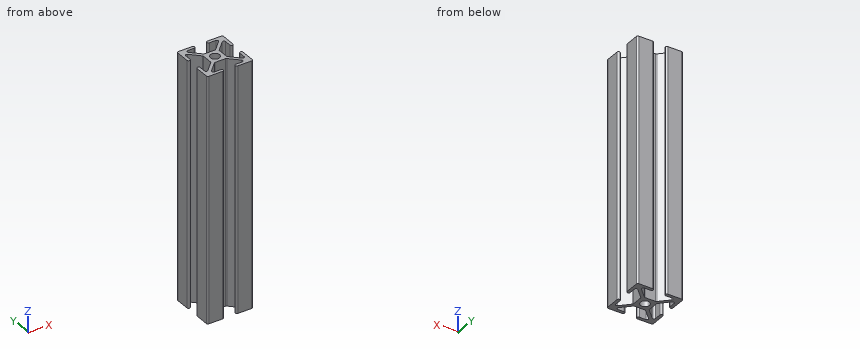
```python
from build123d import *

# Parameters (mm, degrees)
SALIENTE_EXTRUIR1_DEPTH = 190
CROQUIS2_R              = 3
CORTAR_EXTRUIR1_DEPTH   = 192.180542943
CORTAR_EXTRUIR3_DEPTH   = 192.180542943
CROQUIS4_W              = 33.127581221
CROQUIS4_H              = 30
CORTAR_EXTRUIR4_DEPTH   = 38


with BuildPart() as part:
    # Croquis1 → Saliente-Extruir1 (new body)
    with BuildSketch(Plane.XY):
        with BuildLine():
            Line((-14, 15), (14, 15))
            ThreePointArc((14, 15), (14.707106781, 14.707106781), (15, 14))
            Line((15, 14), (15, -14))
            ThreePointArc((15, -14), (14.707106781, -14.707106781), (14, -15))
            Line((14, -15), (-14, -15))
            ThreePointArc((-14, -15), (-14.707106781, -14.707106781), (-15, -14))
            Line((-15, -14), (-15, 14))
            ThreePointArc((-15, 14), (-14.707106781, 14.707106781), (-14, 15))
        make_face()
    extrude(amount=-SALIENTE_EXTRUIR1_DEPTH)

    # Croquis2 → Cortar-Extruir1 (cut, through all)
    with BuildSketch(Plane.XY):
        Circle(CROQUIS2_R)
    extrude(amount=-CORTAR_EXTRUIR1_DEPTH, mode=Mode.SUBTRACT)

    # Croquis3 → Cortar-Extruir3 (cut, through all)
    with BuildSketch(Plane.XY):
        with BuildLine():
            Line((-5.492893219, 4.078679656), (-11.292893219, 9.878679656))
            ThreePointArc((-11.292893219, 9.878679656), (-12.382683432, 10.095452408), (-13, 9.171572875))
            Line((-13, 9.171572875), (-13, 5))
            ThreePointArc((-13, 5), (-14, 4), (-15, 5))
            Line((-15, 5), (-15, -5))
            ThreePointArc((-15, -5), (-14, -4), (-13, -5))
            Line((-13, -5), (-13, -9.171572875))
            ThreePointArc((-13, -9.171572875), (-12.382683432, -10.095452408), (-11.292893219, -9.878679656))
            Line((-11.292893219, -9.878679656), (-5.492893219, -4.078679656))
            ThreePointArc((-5.492893219, -4.078679656), (-5.276120467, -3.754256308), (-5.2, -3.371572875))
            Line((-5.2, -3.371572875), (-5.2, 3.371572875))
            ThreePointArc((-5.2, 3.371572875), (-5.276120467, 3.754256308), (-5.492893219, 4.078679656))
        make_face()
        with BuildLine():
            ThreePointArc((-9.171572875, 13), (-10.095452408, 12.382683432), (-9.878679656, 11.292893219))
            Line((-9.878679656, 11.292893219), (-4.078679656, 5.492893219))
            ThreePointArc((-4.078679656, 5.492893219), (-3.754256308, 5.276120467), (-3.371572875, 5.2))
            Line((-3.371572875, 5.2), (3.371572875, 5.2))
            ThreePointArc((3.371572875, 5.2), (3.754256308, 5.276120467), (4.078679656, 5.492893219))
            Line((4.078679656, 5.492893219), (9.878679656, 11.292893219))
            ThreePointArc((9.878679656, 11.292893219), (10.095452408, 12.382683432), (9.171572875, 13))
            Line((9.171572875, 13), (5, 13))
            ThreePointArc((5, 13), (4, 14), (5, 15))
            Line((5, 15), (-5, 15))
            ThreePointArc((-5, 15), (-4.292893219, 14.707106781), (-4, 14))
            ThreePointArc((-4, 14), (-4.292893219, 13.292893219), (-5, 13))
            Line((-5, 13), (-9.171572875, 13))
        make_face()
        with BuildLine():
            Line((9.878679656, -11.292893219), (4.078679656, -5.492893219))
            ThreePointArc((4.078679656, -5.492893219), (3.754256308, -5.276120467), (3.371572875, -5.2))
            Line((3.371572875, -5.2), (-3.371572875, -5.2))
            ThreePointArc((-3.371572875, -5.2), (-3.754256308, -5.276120467), (-4.078679656, -5.492893219))
            Line((-4.078679656, -5.492893219), (-9.878679656, -11.292893219))
            ThreePointArc((-9.878679656, -11.292893219), (-10.095452408, -12.382683432), (-9.171572875, -13))
            Line((-9.171572875, -13), (-5, -13))
            ThreePointArc((-5, -13), (-4.292893219, -13.292893219), (-4, -14))
            ThreePointArc((-4, -14), (-4.292893219, -14.707106781), (-5, -15))
            Line((-5, -15), (5, -15))
            ThreePointArc((5, -15), (4, -14), (5, -13))
            Line((5, -13), (9.171572875, -13))
            ThreePointArc((9.171572875, -13), (10.095452408, -12.382683432), (9.878679656, -11.292893219))
        make_face()
        with BuildLine():
            ThreePointArc((13, 9.171572875), (12.382683432, 10.095452408), (11.292893219, 9.878679656))
            Line((11.292893219, 9.878679656), (5.492893219, 4.078679656))
            ThreePointArc((5.492893219, 4.078679656), (5.276120467, 3.754256308), (5.2, 3.371572875))
            Line((5.2, 3.371572875), (5.2, -3.371572875))
            ThreePointArc((5.2, -3.371572875), (5.276120467, -3.754256308), (5.492893219, -4.078679656))
            Line((5.492893219, -4.078679656), (11.292893219, -9.878679656))
            ThreePointArc((11.292893219, -9.878679656), (12.382683432, -10.095452408), (13, -9.171572875))
            Line((13, -9.171572875), (13, -5))
            ThreePointArc((13, -5), (14, -4), (15, -5))
            Line((15, -5), (15, 5))
            ThreePointArc((15, 5), (14, 4), (13, 5))
            Line((13, 5), (13, 9.171572875))
        make_face()
    extrude(amount=-CORTAR_EXTRUIR3_DEPTH, mode=Mode.SUBTRACT)

    # Croquis4 → Cortar-Extruir4 (cut)
    with BuildSketch(Plane(origin=(0, 15, 0), x_dir=(1, 0, 0), z_dir=(0, 1, 0))):
        with Locations((-1.56379061, 15)):
            Rectangle(CROQUIS4_W, CROQUIS4_H)
    extrude(amount=-CORTAR_EXTRUIR4_DEPTH, mode=Mode.SUBTRACT)


solid = part.part
```
The model under review builds one solid part; all positions refer to its coordinate system, in mm. Round coordinates to 2 decimals unless told otherwise and drop trailing zeros. Loops run counter-clockwise (first coordinate to the right, second up) from the corner with the lowest first, then second, coordinate; pieces in that order, holes last. Notation, with made-up numbers: (-8, 62) -> (-4, 62) arc R29 ccw to (-4, 94) -> close; hole circle Ø4 at (-29.75, -9). An arc over 180 degrees is marked (long way). Answer as a JSON object with one key per item and string values. Group by question number.
1) We need section C-C on y = -7. Write out the cut boundary in (x, z), then the cut area to 3 significant figures.
2) For line 1 (Y direction, x = 6, z = -95); line 2 (X direction, y = -9.5, z = -133.5); line 3 (Y direction, x = 0, z = -104), list the stretches that pass through material, from the lowest coordinate up. Write a range as [from, to].
3) For pin 1 Ø7.5 at (y, z) = (-0.5, -128.5) entering from -X; pin 2 Ø2 at (x, z) = (0, -124) entering from +Y; pin 3 Ø5.5 at (y, z) = (1, -128.5) entering from +X, all flat-tipped, find the tip position at first contact; note any pin that passes through.
4) We need section A-A on y = 0. Write out the cut boundary in (x, z).
Result set:
{
 "1": {"outline": "(-15, -190) -> (-13, -190) -> (-13, -30) -> (-15, -30) -> close; (-8.41, -190) -> (-5.59, -190) -> (-5.59, -30) -> (-8.41, -30) -> close; (5.59, -190) -> (8.41, -190) -> (8.41, -30) -> (5.59, -30) -> close; (13, -190) -> (15, -190) -> (15, -30) -> (13, -30) -> close", "area": "1,550 mm²"},
 "2": {"line 1": "[-15, -13], [-7.41, -4.59], [4.59, 7.41], [13, 15]", "line 2": "[-15, -12.94], [-10.91, -8.09], [8.09, 10.91], [12.94, 15]", "line 3": "[-5.2, -3], [3, 5.2]"},
 "3": {"pin 1": "x = -14.66", "pin 2": "y = 5.2", "pin 3": "x = 5.27"},
 "4": {"outline": "(-5.2, -190) -> (-3, -190) -> (-3, -30) -> (-5.2, -30) -> close; (3, -190) -> (5.2, -190) -> (5.2, -30) -> (3, -30) -> close"}
}
